from build123d import *

# Parameters (mm, degrees)
SKETCH_1_R      = 2
EXTRUDE_1_DEPTH = 1.5
FILLET_1_R      = 3


with BuildPart() as part:
    # ｽｹｯﾁ1 → ﾎﾞｽ - 押し出し1 (new body)
    # profile 1 of 2: a face of its own
    with BuildSketch(Plane.XY):
        Polygon((-9.402488121, -2.740817625), (5.495827016, -17.259182375), (17.5, -4.940856231), (17.5, 17.259182375), (-17.5, 17.259182375), (-17.5, 5.150184139), align=None)
        with Locations((5.404503628, -10.188704312)):
            Circle(SKETCH_1_R, mode=Mode.SUBTRACT)
        with Locations((-12.5, 7.259182375)):
            Circle(SKETCH_1_R, mode=Mode.SUBTRACT)
        with Locations((12.5, 7.259182375)):
            Circle(SKETCH_1_R, mode=Mode.SUBTRACT)
    # profile 2 of 2: a face of its own
    with BuildSketch(Plane.XY):
        Polygon((-17.5, 5.150184139), (-17.5, -2.740817625), (-9.402488121, -2.740817625), align=None)
    extrude(amount=EXTRUDE_1_DEPTH)

    # ﾌｨﾚｯﾄ1
    fillet_1_edges = [part.edges().sort_by_distance(p)[0] for p in [
        (-9.402488121, -2.740817625, 0.75),
        (-17.5, -2.740817625, 0.75),
        (-17.5, 17.259182375, 0.75),
        (17.5, 17.259182375, 0.75),
        (17.5, -4.940856231, 0.75),
        (5.495827016, -17.259182375, 0.75),
    ]]
    fillet(fillet_1_edges, radius=FILLET_1_R)


solid = part.part
Could you check a few things on this model? Use its own coordinates, in mm. A direction names the side the tool comes from. Give positions to 0.01 mm unless a question says otherwise; leave off trailing zeros. Order: outer loops, then holes, each group sorted by start corner. A loop starts at its lowest first (then second) coordinate and runs counter-clockwise, first axis right, second up. Notation, with made-up numbers: (89.25, -39) -> (98.25, -39) arc R11 ccw to (98.25, -35) -> close; hole circle Ø8 at (-13.5, 11.25). An arc over 180 degrees is marked (long way). Return JSON: item names as keys, results as strings.
1. Imagine slicing it at A-A on x = -12.5. List the corners of the cut face in (y, z) for me, then the cut area to 3 significant figures.
Answer list:
{"outline": "(-2.74, 0) -> (5.26, 0) -> (5.26, 1.5) -> (-2.74, 1.5) -> close; (9.26, 0) -> (17.26, 0) -> (17.26, 1.5) -> (9.26, 1.5) -> close", "area": "24.0 mm2"}
2. Imagine slicing it at B-B on y = 6. List the corners of the cut face in (x, z) for me.
Answer list:
{"outline": "(-17.5, 0) -> (-14.05, 0) -> (-14.05, 1.5) -> (-17.5, 1.5) -> close; (-10.95, 0) -> (10.95, 0) -> (10.95, 1.5) -> (-10.95, 1.5) -> close; (14.05, 0) -> (17.5, 0) -> (17.5, 1.5) -> (14.05, 1.5) -> close"}
3. On a 3-axis mill with a long thin cutter (end or side, diameter ignored), from which of +Z, -Z, +X, -X, +Y, -Y can I reach the whole of each face in a straight line? I mean faces 4 (the flat face through (-13, -2.741, 1)), 5 (the cylindrical face through (17.3, -4.8, 0.8)). Say none if no direction works.
Answer list:
{"face 4": "+Z, -Z, -X, -Y", "face 5": "+Z, -Z, +X, -Y"}
4. I need wall thicknesses on line 1 (Y direction, x = -12.5, z = 1.1); line 2 (X direction, y = 8, z = 0.4); line 3 (X direction, y = 7, z = 0.15). Which ranges of each line are inside material? Lowest first, please. Write a range as from..to.
Answer list:
{"line 1": "y = -2.74..5.26, 9.26..17.26", "line 2": "x = -17.5..-14.36, -10.64..10.64, 14.36..17.5", "line 3": "x = -17.5..-14.48, -10.52..10.52, 14.48..17.5"}
5. For pin 1 Ø6.5 at (x, y) = (5.4, -10.19) entering from -Z, with a flat end and sliding along its axis, tell me the tip position at first contact or that it passes through.
Answer list:
{"pin 1": "stops at z = 0"}
6. Imagine slicing it at D-D on x = 12.5. List the corners of the cut face in (y, z) for me, then the cut area to 3 significant figures.
Answer list:
{"outline": "(-10.07, 0) -> (5.26, 0) -> (5.26, 1.5) -> (-10.07, 1.5) -> close; (9.26, 0) -> (17.26, 0) -> (17.26, 1.5) -> (9.26, 1.5) -> close", "area": "35.0 mm2"}
7. Thinking about a two-plate mould opening in Y: for faces 1 (the cylindrical face through (6.33, -11.96, 0.74)), 2 (the flat face through (-2.67, -9.3, 0.74)), 3 (the cylindrical face through (-16.6, 16.4, 0.8)), which applies, pulls with the +Y half, pulls with the -Y half, needs draft (parallel to the pull), parting line crosses it, or undercut?
Answer list:
{"face 1": "undercut", "face 2": "pulls with the -Y half", "face 3": "pulls with the +Y half"}
8. Imagine slicing it at C-C on z = 0.65. List the corners of the cut face in (x, y) for me.
Answer list:
{"outline": "(-17.5, 0.26) arc R3 ccw to (-14.5, -2.74) -> (-10.62, -2.74) arc R3 cw to (-8.53, -3.59) -> (3.35, -15.17) arc R3 ccw to (7.59, -15.11) -> (16.65, -5.81) arc R3 ccw to (17.5, -3.72) -> (17.5, 14.26) arc R3 ccw to (14.5, 17.26) -> (-14.5, 17.26) arc R3 ccw to (-17.5, 14.26) -> close; hole circle Ø4 at (-12.5, 7.26); hole circle Ø4 at (5.4, -10.19); hole circle Ø4 at (12.5, 7.26)"}
